```python
from build123d import *

# Parameters (mm, degrees)
SKETCH1_R           = 95.25
BOSS_EXTRUDE1_DEPTH = 19.05
SKETCH2_R           = 31.75
CUT_EXTRUDE1_DEPTH  = 10.16
SKETCH3_R           = 56.515
CUT_EXTRUDE2_DEPTH  = 27.94
SKETCH4_R           = 3.175
CUT_EXTRUDE3_DEPTH  = 19.05
CIRPATTERN1_COUNT   = 3


with BuildPart() as part:
    # Sketch1 → Boss-Extrude1 (new body, symmetric)
    with BuildSketch(Plane(origin=(0, 0, 0), x_dir=(1, 0, 0), z_dir=(0, 1, 0))):
        Circle(SKETCH1_R)
    extrude(amount=BOSS_EXTRUDE1_DEPTH, both=True)

    # Sketch2 → Cut-Extrude1 (cut)
    with BuildSketch(Plane(origin=(0, 19.05, 0), x_dir=(1, 0, 0), z_dir=(0, 1, 0))):
        Circle(SKETCH2_R)
    extrude(amount=-CUT_EXTRUDE1_DEPTH, mode=Mode.SUBTRACT)

    # Sketch3 → Cut-Extrude2 (cut)
    with BuildSketch(Plane.XZ.offset(19.05)):
        Circle(SKETCH3_R)
    extrude(amount=-CUT_EXTRUDE2_DEPTH, mode=Mode.SUBTRACT)

    # Sketch4 → Cut-Extrude3 (cut)
    with BuildSketch(Plane.XZ.offset(19.05)):
        with Locations((-76.2, 0)):
            Circle(SKETCH4_R)
    cut_extrude3 = extrude(amount=-CUT_EXTRUDE3_DEPTH, mode=Mode.SUBTRACT)

    # CirPattern1: Cut-Extrude3 ×3 about axis
    cirpattern1_axis = Axis((0, 0, 0), (0, 1, 0))
    for i in range(1, CIRPATTERN1_COUNT):
        add(cut_extrude3.rotate(cirpattern1_axis, i * 360 / CIRPATTERN1_COUNT), mode=Mode.SUBTRACT)


solid = part.part
```
Work out the finished part from the listing and answer in its coordinate system (mm). A direction names the side the tool comes from. Coordinates: 2 decimals unless noted, no trailing zeros. Loops run counter-clockwise (first coordinate to the right, second up) from the corner with the lowest first, then second, coordinate; pieces in that order, holes last.
1) Section A-A (x = 0) is taken. Give the vertices of the cut face in (y, z) (3 decimals), plus the area to 3 significant figures.
Results:
outline: (-19.05, -95.25) - (19.05, -95.25) - (19.05, -31.75) - (8.89, -31.75) - (8.89, -56.515) - (-19.05, -56.515) - close; (-19.05, 56.515) - (8.89, 56.515) - (8.89, 31.75) - (19.05, 31.75) - (19.05, 95.25) - (-19.05, 95.25) - close
area: 3,450 mm2
2) Section B-B (z = 0) is taken. Give the vertices of the cut face in (x, y) (3 decimals), plus the area to 3 significant figures.
Results:
outline: (-95.25, -19.05) - (-79.375, -19.05) - (-79.375, 0) - (-73.025, 0) - (-73.025, -19.05) - (-56.515, -19.05) - (-56.515, 8.89) - (-31.75, 8.89) - (-31.75, 19.05) - (-95.25, 19.05) - close; (31.75, 8.89) - (56.515, 8.89) - (56.515, -19.05) - (95.25, -19.05) - (95.25, 19.05) - (31.75, 19.05) - close
area: 3,330 mm2
3) Section D-D (z = 44) is taken. Give the vertices of the cut face in (x, y), plus the area to 3 significant figures.
Results:
outline: (-84.48, -19.05) - (-35.47, -19.05) - (-35.47, 8.89) - (35.47, 8.89) - (35.47, -19.05) - (84.48, -19.05) - (84.48, 19.05) - (-84.48, 19.05) - close
area: 4,460 mm2
4) Flat-ended cylindrical pins translate along their axes: pin 1 (5 mm diameter, centred on x = -75, z = -0.5, fed in from -Y); pin 2 (10 mm diameter, centred on x = 25, z = 44.5, fed in from -Y); pin 3 (10 mm diameter, centred on x = 72, y = -5, fed in from +Z); pin 4 (1.5 mm diameter, centred on x = -42, y = -1, fed in from -Z). Find the tip coordinate at first contact, or state that the pin passes through.
Results:
pin 1: stops at y = -19.05
pin 2: stops at y = 8.89
pin 3: stops at z = 67.7
pin 4: stops at z = -85.85
5) Section C-C (y = -16) is taken. Give the number of separate pieces and of enclosed holes in the cut face, plus the area to 3 significant figures.
Results:
separate pieces: 1
enclosed holes: 4
area: 18,400 mm2
6) For a pull along Z with two mould halves and no side action, classify faces 3 (the cylindrical face through (-75.587, 0.267, 57.958)), 4 (the cylindrical face through (-44.848, -5.276, -34.388)), 5 (the flat face through (-23, 19.05, -23)) as +Z half, -Z half, draft (parallel to the pull), parting line (faces both ways), or undercut.
Results:
face 3: parting line
face 4: undercut
face 5: draft
7) For faces 1 (the cylindrical face through (37.687, -9.658, -62.843)), 2 (the flat face through (41, -19.05, 41)), determine the directions among +Z, -Z, +X, -X, +Y, -Y from which every point of the face is accessible in a straight line to the end or side of a thin tool.
Results:
face 1: -Y
face 2: +Z, -Z, +X, -X, -Y
8) Consider probe 1 along X at (y, z) = (13, 0); probe 2 along Z at (x, y) = (0, -11) (3 decimals); probe 3 along Y at (x, z) = (-55.5, 4). Determine where each line is inside the solid, lowest interval first.
Results:
probe 1: x = -95.25 to -31.75, 31.75 to 95.25
probe 2: z = -95.25 to -56.515, 56.515 to 95.25
probe 3: y = 8.89 to 19.05
